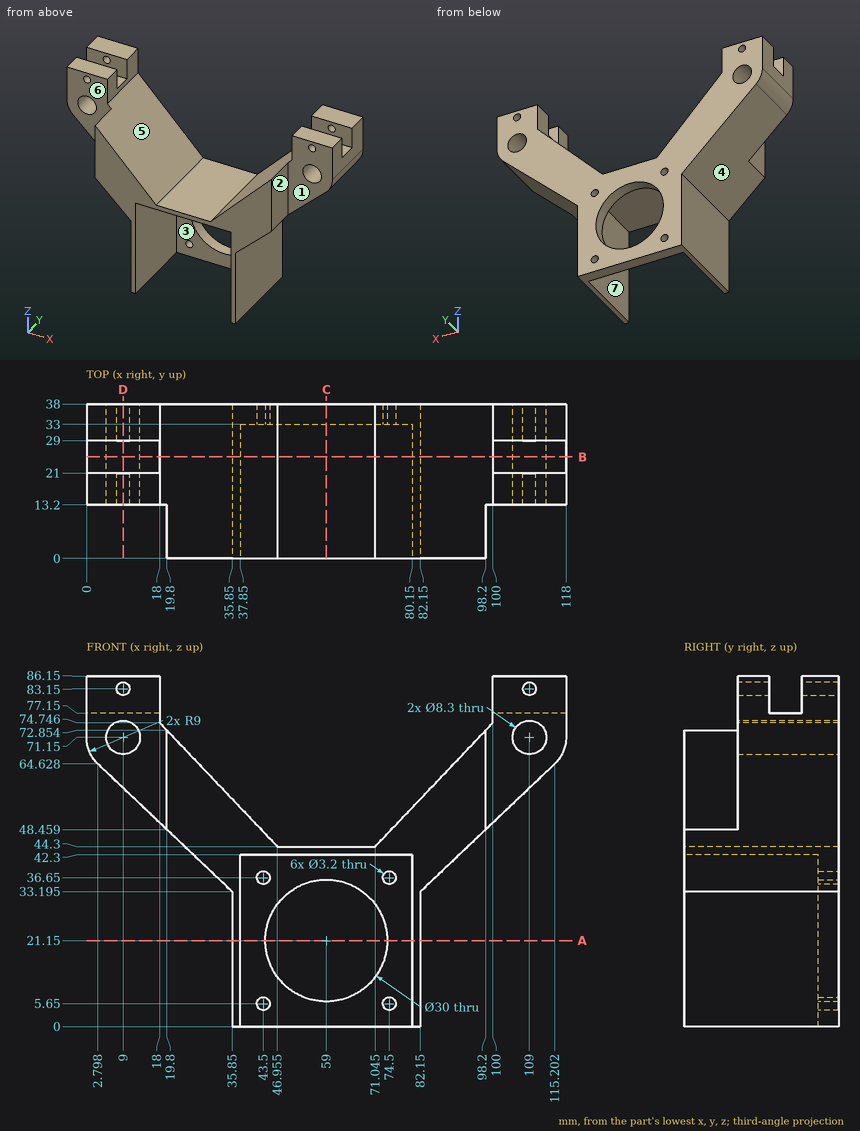
Geometry check sheet. Reference: drawing and pictorial views, mm from the part's lowest x, y, z. A direction names the side the tool comes from. Give positions to 0.01 mm unless a question says otherwise; leave off trailing zeros. Order: outer loops, then holes, each group sorted by start corner. A loop starts at its lowest first (then second) coordinate and runs counter-clockwise, first axis right, second up. Notation, with made-up numbers: (-14, 35) - (30, 35) arc R6 cw to (30, 40) - close; hole circle Ø7 at (27, 34). An arc over 180 degrees is marked (long way). Answer as CSV lines item,"result". Start each with the question number.
Item 1: Gauge pin test, flat ends, axial feed: pin 1 (10 mm diameter, centred on x = 73, z = 49.5, fed in from -Y); pin 2 (4 mm diameter, centred on x = 24, y = 26, fed in from -Z); pin 3 (2.5 mm diameter, centred on x = 74.5, z = 5.65, fed in from -Y); pin 4 (3 mm diameter, centred on y = 24.5, z = 53, fed in from -X). Record the tip position at first contact, or that the pin passes through.
Item 2: Access from +Z, -Z, +X, -X, +Y, -Y to the whole of each face (thin tool, end or side, straight path). Record for the marked faces 5, 6 and 7.
Item 3: Section check B-B, the plane y = 25. State how many separate pieces and enclosed holes the cut face has, plus the area to 3 significant figures.
Item 4: Mould release check, pull along X, two halves, no side actions. Record for the marked faces 1, 2, 3 and 4: released by +X, released by -X, zero draft, split by the parting line, or undercut.
Item 5: Section check C-C, the plane x = 59. Record the boundary of the cut face in (y, z).
Item 6: Section check A-A, the plane z = 21.15. Record the boundary of the cut face in (x, y).
Item 7: Material ranges on L1, parallel to X at y = 34.9, z = 21.15; L2, parallel to X at y = 32.75, z = 83.15; L3, parallel to Y at x = 17, z = 79, recorded low to high.
Item 8: Section check D-D, the plane x = 9. Record the boundary of the cut face in (y, z).
Filled in:
1,pin 1,"y = 0"
1,pin 2,"z = 42.56"
1,pin 3,"through"
1,pin 4,"x = 13.45"
2,face 5,"+Z, +Y, -Y"
2,face 6,"+Z, -Z, -X, -Y"
2,face 7,"-Z, -Y"
3,separate pieces,"1"
3,enclosed holes,"2"
3,area,"1,790 mm^2"
4,face 1,"zero draft"
4,face 2,"released by +X"
4,face 3,"undercut"
4,face 4,"released by -X"
5,outline,"(0, 42.3) - (33, 42.3) - (33, 36.15) - (38, 36.15) - (38, 44.3) - (0, 44.3) - close; (33, 0) - (38, 0) - (38, 6.15) - (33, 6.15) - close"
6,outline,"(35.85, 0) - (37.85, 0) - (37.85, 33) - (44, 33) - (44, 38) - (35.85, 38) - close; (74, 33) - (80.15, 33) - (80.15, 0) - (82.15, 0) - (82.15, 38) - (74, 38) - close"
7,L1,"35.85 to 44, 74 to 82.15"
7,L2,"0 to 7.4, 10.6 to 18, 100 to 107.4, 110.6 to 118"
7,L3,"13.2 to 21, 29 to 38"
8,outline,"(13.2, 58.73) - (38, 58.73) - (38, 67) - (13.2, 67) - close; (13.2, 75.3) - (38, 75.3) - (38, 81.55) - (29, 81.55) - (29, 77.15) - (21, 77.15) - (21, 81.55) - (13.2, 81.55) - close; (13.2, 84.75) - (21, 84.75) - (21, 86.15) - (13.2, 86.15) - close; (29, 84.75) - (38, 84.75) - (38, 86.15) - (29, 86.15) - close"
